Can you work these out from the drawing? Everything is in mm from the part's minimum corner. A direction names the side the tool comes from. Give positions to 0.01 mm unless a question says otherwise; leave off trailing zeros. Write each loop counter-clockwise with the first axis right and the second up, starting at its lowest first coordinate (ties: lowest second). Pieces come first, ordered by that corner, then holes. Notation, with made-up numbers: (-1.75, 49) - (19.25, 49) arc R12 cw to (19.25, 60) - close; hole circle Ø3 at (30.25, 21). An arc over 180 degrees is marked (long way). Use a Markdown table: item, result. Add a question column.
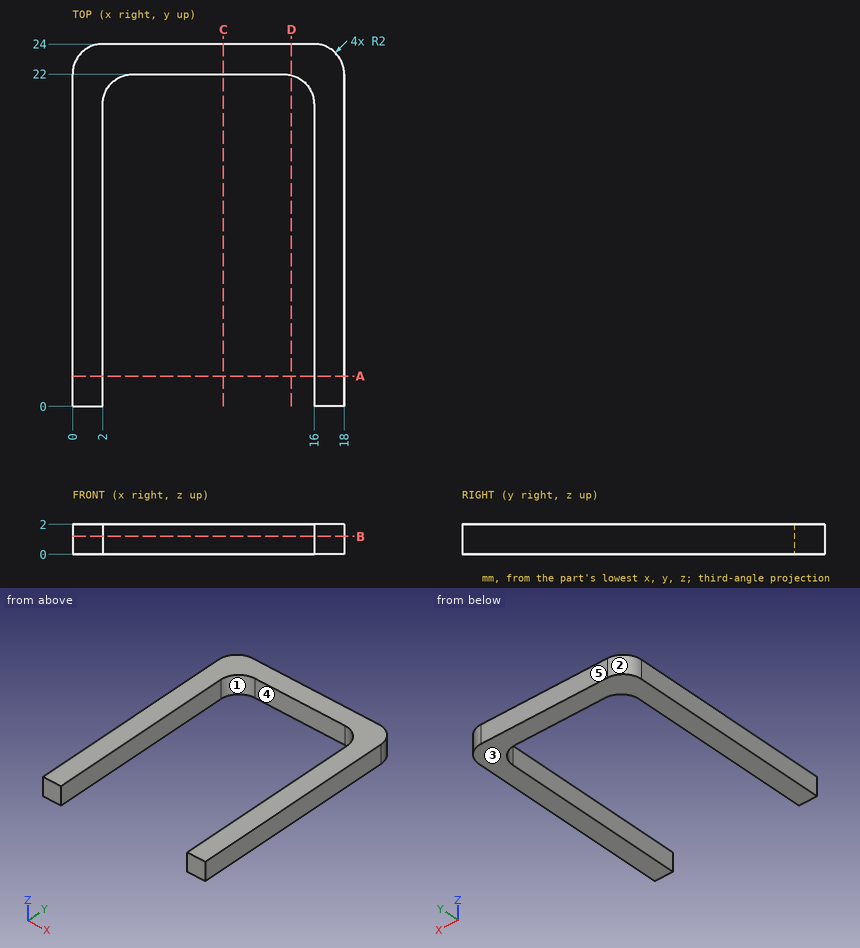
Q1. If I drill on probe 1 along X at (y, z) = (9.25, 0.15); probe 2 along Y at (x, z) = (4.25, 0.35); probe 3 along X at (y, z) = (21.5, 0.1), over which ranges is the centre line in solid material (lowest first)? Write a range as [from, to].
Q2. If we mould it in two halves opening along X, with no side actions, what happens to the marked faces 1, 2 and 3? For each: released by +X, released by -X, zero draft, split by the parting line, or undercut.
Q3. Suppose I cut it at A-A (y = 2). Please give me the cut outline in (x, z), and give its area (3 significant figures).
Q4. Suppose I cut it at D-D (x = 14.5). Please give me the cut outline in (y, z).
Q5. Suppose I cut it at B-B (z = 1.2). Please give me the cut outline in (x, y).
Q6. Suppose I cut it at C-C (x = 10). Please give me the cut outline in (y, z).
Q7. On a 3-axis mill with a long thin cutter (end or side, diameter ignored), from which of +Z, -Z, +X, -X, +Y, -Y can I reach the whole of each face in a straight line? I mean the marked faces 4 and 5. Say none if no direction works.
Q8. I'm going to push flat-ended pins straight in: P1, Ø1, axis at x = 11, z = 1, coming from the -Y side; P2, Ø5, axis at x = 3.5, y = 6.5, coming from the -Z side. Where does each tip first touch, or does it pass through?
Derived:
| question | item | result |
|---|---|---|
| 1 | probe 1 | [0, 2], [16, 18] |
| 1 | probe 2 | [22, 24] |
| 1 | probe 3 | [0, 2.68], [15.32, 18] |
| 2 | face 1 | undercut |
| 2 | face 2 | released by -X |
| 2 | face 3 | zero draft |
| 3 | outline | (0, 0) - (2, 0) - (2, 2) - (0, 2) - close; (16, 0) - (18, 0) - (18, 2) - (16, 2) - close |
| 3 | area | 8.00 mm² |
| 4 | outline | (21.94, 0) - (24, 0) - (24, 2) - (21.94, 2) - close |
| 5 | outline | (0, 0) - (2, 0) - (2, 20) arc R2 cw to (4, 22) - (14, 22) arc R2 cw to (16, 20) - (16, 0) - (18, 0) - (18, 22) arc R2 ccw to (16, 24) - (2, 24) arc R2 ccw to (0, 22) - close |
| 6 | outline | (22, 0) - (24, 0) - (24, 2) - (22, 2) - close |
| 7 | face 4 | +Z, -Z, -Y |
| 7 | face 5 | +Z, -Z, +X, -X, +Y |
| 8 | P1 | y = 22 |
| 8 | P2 | z = 0 |
